Can you work these out from the drawing? Everything is in mm from the part's minimum corner. Coordinates: 2 decimals unless noted, no trailing zeros. Loops run counter-clockwise (first coordinate to the right, second up) from the corner with the lowest first, then second, coordinate; pieces in that order, holes last.
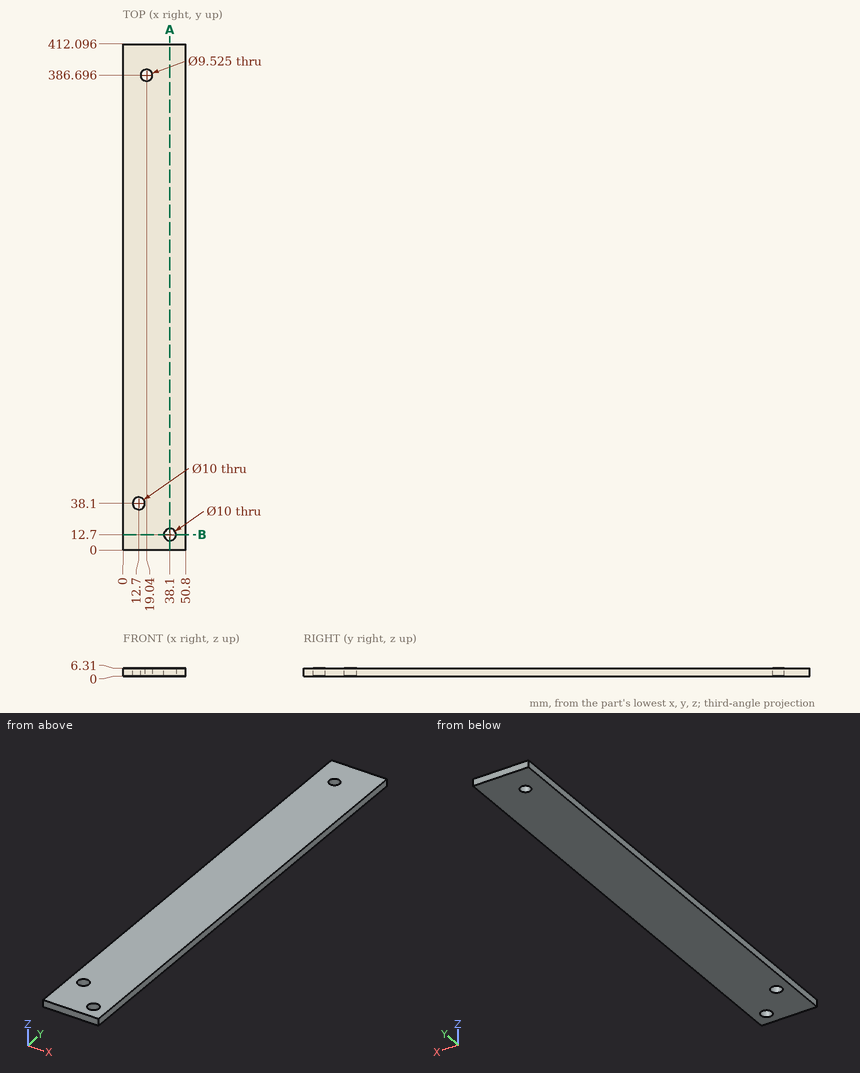
1. I want a section at B-B (y = 12.7). Please give me the cut outline in (x, z).
2. I need wall thicknesses on line 1 along Y through (x, z) = (38.1, 3.75) (1 decimal); line 2 along Y through (x, z) = (12.7, 3.75) (1 decimal). Which ranges of each line are inside material? Lowest first, please.
3. I want a section at A-A (x = 38.1). Please give me the cut outline in (y, z) (1 decimal).
4. For pin 1 (11.5 mm diameter, centred on x = 12.7, y = 38.1, fed in from +Z); pin 2 (9 mm diameter, centred on x = 38.1, y = 12.7, fed in from -Z), each with a flat end and sliding along its axis, tell me the tip position at first contact or that it passes through.
Response values:
1. outline: (0, 0) - (33.1, 0) - (33.1, 6.31) - (0, 6.31) - close; (43.1, 0) - (50.8, 0) - (50.8, 6.31) - (43.1, 6.31) - close
2. line 1: y = 0 to 7.7, 17.7 to 412.1
2. line 2: y = 0 to 33.1, 43.1 to 412.1
3. outline: (0, 0) - (7.7, 0) - (7.7, 6.3) - (0, 6.3) - close; (17.7, 0) - (412.1, 0) - (412.1, 6.3) - (17.7, 6.3) - close
4. pin 1: stops at z = 6.31
4. pin 2: passes through
